Here's how the part is built. I have some questions about the finished solid (model axes, mm). Face numbers are marked on the shaded views. A direction names the side the tool comes from. Coordinates: 2 decimals unless noted, no trailing zeros. Write each loop counter-clockwise with the first axis right and the second up, starting at its lowest first coordinate (ties: lowest second). Pieces come first, ordered by that corner, then holes. Notation, with made-up numbers: (32, -21) -> (55, -21) arc R22 ccw to (55, -9) -> close; hole circle Ø7 at (57.5, 87.25). An arc over 180 degrees is marked (long way). Put each result on its own line as item: value.
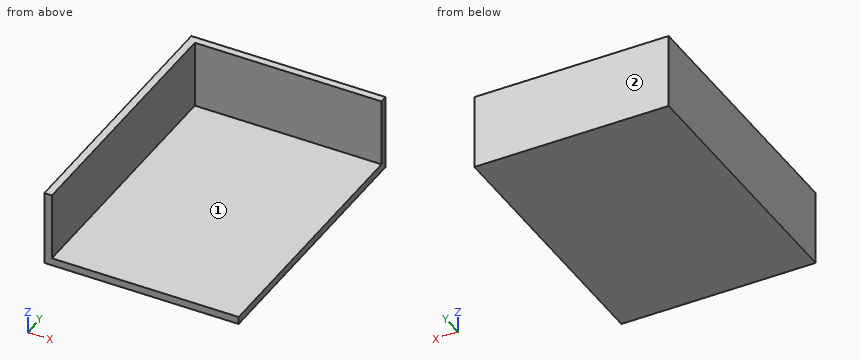
```python
from build123d import *

# Parameters (mm, degrees)
F2_W     = 65.475806
F2_H     = 91.311798
F0_DEPTH = 25.4
F1_T     = -2.54


with BuildPart() as f0:
    # F2 (on Top) → F0 (new body)
    with BuildSketch(Plane.XY):
        with Locations((16.99128, 32.161951)):
            Rectangle(F2_W, F2_H)
    extrude(amount=F0_DEPTH)

    # F1
    f1_openings = [f0.faces().sort_by_distance(p)[0] for p in [
        (49.729183, 32.161951, 12.7),
        (16.99128, -13.493948, 12.7),
        (16.99128, 32.161951, 25.4),
    ]]
    offset(amount=F1_T, openings=f1_openings)


solid = f0.part
```
Item 1: Imagine slicing it at B-B on z = 19.75. Write out the boundary of the cut face in (x, y), then the cut area to 3 significant figures.
Output:
outline: (-15.75, -13.49) -> (-13.21, -13.49) -> (-13.21, 75.28) -> (49.73, 75.28) -> (49.73, 77.82) -> (-15.75, 77.82) -> close
area: 392 mm²
Item 2: Imagine slicing it at A-A on y = 53.5. Write out the boundary of the cut face in (x, z), then the cut area to 3 significant figures.
Output:
outline: (-15.75, 0) -> (49.73, 0) -> (49.73, 2.54) -> (-13.21, 2.54) -> (-13.21, 25.4) -> (-15.75, 25.4) -> close
area: 224 mm²
Item 3: Please list where these lines run through material, in increasing order: line 1 along Z through (x, y) = (7, 51); line 2 along Y through (x, z) = (6.5, 17); line 3 along X through (y, z) = (51.5, 22). Write a range as from..to.
Output:
line 1: z = 0..2.54
line 2: y = 75.28..77.82
line 3: x = -15.75..-13.21
Item 4: For P1, Ø7, axis at y = 15, z = 14.5, coming from the +X side; P2, Ø12, axis at x = 10, z = 22, coming from the -Y side, each with a flat end and sliding along its axis, tell me the tip position at first contact or that it passes through.
Output:
P1: stops at x = -13.21
P2: stops at y = 75.28
Item 5: Which directions (+Z, -Z, +X, -X, +Y, -Y) give clear straight access to the entire face, cutting with the end or side of a thin tool? Please do the marked faces 1 and 2.
Output:
face 1: +Z, +X, -Y
face 2: +Z, -Z, +X, -X, +Y
